Build history of the part. All positions in model axes, mm. Face numbers are marked on the shaded views. A direction names the side the tool comes from. Coordinates: 2 decimals unless noted, no trailing zeros. Loops run counter-clockwise (first coordinate to the right, second up) from the corner with the lowest first, then second, coordinate; pieces in that order, holes last.
Item 1: Cut at A-A (z = 33). List the corners of the cut face in (x, y).
Item 2: Flat gauge pins, fed straight in: pin 1 (12 mm diameter, centred on x = -3.5, y = 76, fed in from +Z); pin 2 (1.6 mm diameter, centred on x = 0, y = 77.5, fed in from -Z); pin 3 (2.5 mm diameter, centred on x = -10.5, y = 84, fed in from +Z). Where does each tip first touch, or does it go through?
Item 3: 3-axis set-ups, long thin cutter, end or side, ignore diameter. For the marked faces 4, 5, 6 and 7: which of +Z, -Z, +X, -X, +Y, -Y reach the whole face in a straight line?
Item 4: Cut at B-B (y = 120). List the corners of the cut face in (x, z), and give its area (3 significant figures).
Item 5: Mould opens along Y. For the marked faces 1, 2 and 3 say: released by +Y, released by -Y, zero draft, split by the parting line, or undercut.
Item 6: Drill centre lines: line 1 along Y through (x, z) = (11, 30); line 2 along Y through (x, z) = (-10, 29.5); line 3 along Z through (x, y) = (-18, 115). Where is each one in solid material? Low to high.
from build123d import *

# Parameters (mm, degrees)
PAD003_DEPTH    = 20
SKETCH006_R     = 4.5
SKETCH006_R_2   = 1.1
POCKET001_DEPTH = 112.6287098757
SKETCH007_R     = 2.5
SKETCH007_R_2   = 1
PAD004_DEPTH    = 12
FILLET002_R     = 2
SKETCH008_R     = 1
POCKET002_DEPTH = 5
CHAMFER_SIZE    = 1


with BuildPart() as part:
    # Sketch005 → Pad003 (new body, symmetric)
    with BuildSketch(Plane.YZ):
        Polygon((143.6765268423, 41.2666689085), (155.3233838719, 84.7333310915), (151.4596805668, 85.7686072719), (139.9764644611, 42.9126613312), (129.0082348028, 26), (84.4999553571, 26), (64.4999553571, 26), (52.8265628624, 8), (39, 8), (39, 4), (47, 4), (55, 4), (66.6733924947, 22), (131.1816719404, 22), align=None)
    extrude(amount=PAD003_DEPTH, both=True)

    # Sketch006 (on Face8 of Pad003) → Pocket001 (cut, through all)
    with BuildSketch(Plane(origin=(0, 123.7353572805, -33.1547890585), x_dir=(0, 0.2588190451, 0.9659258263), z_dir=(0, 0.9659258263, -0.2588190451))):
        with Locations((99.5467627446, 0)):
            Circle(SKETCH006_R)
        with Locations((99.6467627446, 10.5)):
            Circle(SKETCH006_R_2)
        with Locations((99.6467627446, -10.5)):
            Circle(SKETCH006_R_2)
        with Locations((87.1467627446, -10.5)):
            Circle(SKETCH006_R_2)
        with Locations((87.1467627446, 10.5)):
            Circle(SKETCH006_R_2)
    extrude(amount=-POCKET001_DEPTH, mode=Mode.SUBTRACT)

    # Sketch007 (on Face16 of Pocket001) → Pad004 (join)
    with BuildSketch(Plane(origin=(0, 0, 26), x_dir=(0, -1, 0), z_dir=(0, 0, 1))):
        Polygon((-80.4999553571, 20), (-88.4999553571, 20), (-88.4999553571, -20), (-80.4999553571, -20), (-74.4999553571, -9.6076951546), (-74.4999553571, 9.6076951546), align=None)
        with Locations((-84.4999553571, -11.25)):
            Circle(SKETCH007_R, mode=Mode.SUBTRACT)
        with Locations((-84.4999553571, 11.25)):
            Circle(SKETCH007_R, mode=Mode.SUBTRACT)
        with Locations((-77.4999553571, 0)):
            Circle(SKETCH007_R_2, mode=Mode.SUBTRACT)
    extrude(amount=PAD004_DEPTH)

    # Fillet002
    fillet002_edges = [part.edges().sort_by_distance(p)[0] for p in [
        (0, 139.976464, 42.912661),
        (0, 52.826563, 8),
        (0, 129.008235, 26),
        (0, 64.499955, 26),
        (0, 39, 8),
        (0, 143.676527, 41.266669),
        (0, 131.181672, 22),
        (0, 66.673392, 22),
    ]]
    fillet(fillet002_edges, radius=FILLET002_R)

    # Sketch008 (on Face8 of Pad004) → Pocket002 (cut)
    with BuildSketch(Plane.YX.offset(-4)):
        with Locations((44.3333333333, 15)):
            Circle(SKETCH008_R)
        with Locations((44.3333333333, -15)):
            Circle(SKETCH008_R)
        with Locations((49.6666666667, 0)):
            Circle(SKETCH008_R)
    extrude(amount=-POCKET002_DEPTH, mode=Mode.SUBTRACT)

    # Chamfer
    chamfer_edges = [part.edges().sort_by_distance(p)[0] for p in [
        (15, 43.333333, 8),
        (0, 48.666667, 8),
        (-15, 43.333333, 8),
    ]]
    chamfer(chamfer_edges, length=CHAMFER_SIZE)


solid = part.part
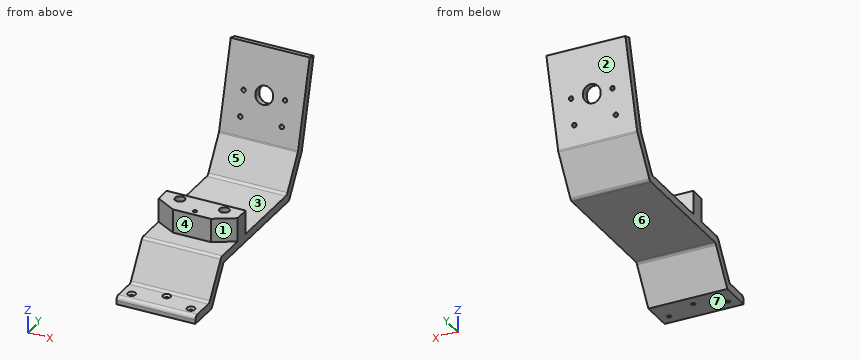
Filled sheet:
1. outline: (-20, 80.5) - (-9.61, 74.5) - (9.61, 74.5) - (20, 80.5) - (20, 88.5) - (-20, 88.5) - close; (-20, 133.55) - (20, 133.55) - (20, 138.32) - (-20, 138.32) - close; hole circle Ø5 at (-11.25, 84.5); hole circle Ø2 at (0, 77.5); hole circle Ø5 at (11.25, 84.5)
2. pin 1: stops at z = 38
2. pin 2: stops at z = 22
2. pin 3: stops at z = 26
3. face 4: +Z, +X, -X, -Y
3. face 5: +Z, +X, -X
3. face 6: -Z, +X, -X, +Y
3. face 7: -Z, +X, -X, +Y, -Y
4. outline: (-20, 22) - (20, 22) - (20, 26) - (-20, 26) - close
4. area: 160 mm2
5. face 1: released by -Y
5. face 2: released by +Y
5. face 3: undercut
6. line 1: y = 75.3 to 82.01, 86.99 to 88.5, 131.6 to 136.37
6. line 2: y = 74.73 to 82.33, 86.67 to 88.5, 131.28 to 136.05
6. line 3: z = 22 to 26
